Read the model definition and answer for the solid it produces. Units are mm, in the model's axes. Face numbers are marked on the shaded views. A direction names the side the tool comes from. Give positions to 0.01 mm unless a question says otherwise; leave off trailing zeros. Loops run counter-clockwise (first coordinate to the right, second up) from the corner with the lowest first, then second, coordinate; pieces in that order, holes last. Notation, with made-up numbers: (47.25, 20) -> (86.25, 20) arc R24 cw to (86.25, 46) -> close; hole circle Ø9 at (66.5, -2). An arc over 180 degrees is marked (long way). One line per item, written item: value. Start each with the question number.
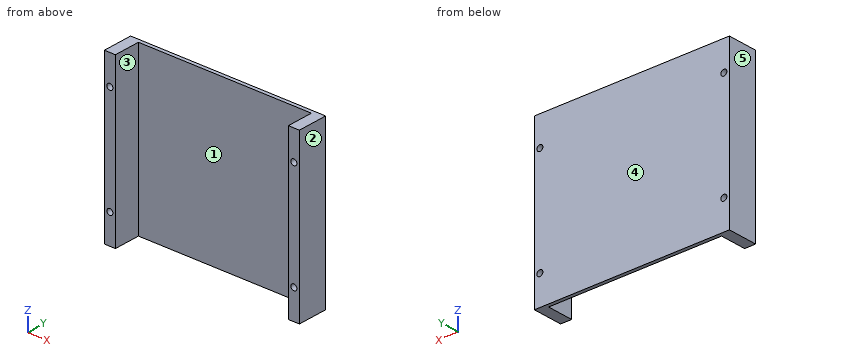
Autodesk Inventor part; units mm, degrees
ref_plane "YZ Plane" through (0, 0, 0) normal (1, 0, 0) x (0, 1, 0)
ref_plane "XZ Plane" through (0, 0, 0) normal (0, 1, 0) x (-1, 0, 0)
ref_plane "XY Plane" through (0, 0, 0) normal (0, 0, 1) x (1, 0, 0)
sketch "Sketch1" plane through (0, 0, 0) normal (0, 0, 1) x (1, 0, 0)
  line L0 (0, 26.035) -> (-84.1883, 26.035)
  line L1 (-84.1883, 26.035) -> (-84.1883, 0)
  line L2 (-84.1883, 0) -> (-74.6633, 0)
  line L3 (-74.6633, 0) -> (-74.6633, 22.86)
  line L4 (-74.6633, 22.86) -> (0, 22.86)
  line L5 (0, 0) -> (0, 26.035) construction
  line L6 (0, 26.035) -> (84.1883, 26.035)
  line L7 (84.1883, 26.035) -> (84.1883, 0)
  line L8 (84.1883, 0) -> (74.6633, 0)
  line L9 (74.6633, 0) -> (74.6633, 22.86)
  line L10 (74.6633, 22.86) -> (0, 22.86)
  dimension "d0" = 22.86
  dimension "d1" = 3.175
  dimension "d2" = 9.525
  dimension "d3" = 74.6633
extrude "Extrusion1" add sketch "Sketch1" along normal mid plane 143.1798
sketch "Sketch2" plane through (-84.1883, 0, 71.5899) normal (0, -1, 0) x (1, 0, 0)
  line L0 (0, -143.1798) -> (168.3766, -143.1798) construction
  line L1 (4.7625, -143.1798) -> (4.7625, -0.1575) construction
  line L2 (0, 0) -> (9.525, 0)
  point P0 (84.1883, -71.5899)
  point P1 (4.7625, -117.7798)
  point P2 (4.7625, -25.4)
  dimension "d6" = 4.7625
  dimension "d7" = 25.4
  dimension "d8" = 25.4
hole "Hole1" at (-79.4258, 0, -46.1899) at (-79.4258, 0, 46.1899) direction (0, 1, 0) diameter 5.1054 end through all
mirror "Mirror1" about plane through (0, 0, 0) normal (1, 0, 0) of "Hole1"
sketch "Sketch3" plane through (-84.1883, 26.035, 71.5899) normal (0, 1, 0) x (1, 0, 0)
  line L0 (11.1125, 0) -> (157.2641, 0) construction
  line L1 (157.2641, 0) -> (157.2641, 143.1798) construction
  line L2 (157.2641, 143.1798) -> (11.1125, 143.1798) construction
  line L3 (11.1125, 143.1798) -> (11.1125, 0) construction
  line L4 (11.1125, 0) -> (157.2641, 143.1798) construction
  line L5 (157.2641, 0) -> (11.1125, 143.1798) construction
  line L6 (51.9303, 1.2954) -> (83.4263, 1.2954)
  line L7 (83.4263, 1.2954) -> (83.4263, 9.9314)
  line L8 (83.4263, 9.9314) -> (51.9303, 9.9314)
  line L9 (51.9303, 9.9314) -> (51.9303, 1.2954)
  line L10 (51.9303, 1.2954) -> (83.4263, 9.9314) construction
  line L11 (83.4263, 1.2954) -> (51.9303, 9.9314) construction
  line L12 (168.3766, 0) -> (0, 0)
  line L13 (84.9503, 1.2954) -> (116.4463, 1.2954)
  line L14 (116.4463, 1.2954) -> (116.4463, 9.9314)
  line L15 (116.4463, 9.9314) -> (84.9503, 9.9314)
  line L16 (84.9503, 9.9314) -> (84.9503, 1.2954)
  line L17 (84.9503, 1.2954) -> (116.4463, 9.9314) construction
  line L18 (116.4463, 1.2954) -> (84.9503, 9.9314) construction
  line L19 (123.5075, 2.8702) -> (145.4785, 2.8702)
  line L20 (145.4785, 2.8702) -> (145.4785, 20.6502)
  line L21 (145.4785, 20.6502) -> (123.5075, 20.6502)
  line L22 (123.5075, 20.6502) -> (123.5075, 2.8702)
  line L23 (123.5075, 2.8702) -> (145.4785, 20.6502) construction
  line L24 (145.4785, 2.8702) -> (123.5075, 20.6502) construction
  line L25 (15.2273, 15.1892) -> (24.7523, 15.1892)
  line L26 (24.7523, 15.1892) -> (24.7523, 92.4052)
  line L27 (24.7523, 92.4052) -> (15.2273, 92.4052)
  line L28 (15.2273, 92.4052) -> (15.2273, 15.1892)
  line L29 (15.2273, 15.1892) -> (24.7523, 92.4052) construction
  line L30 (24.7523, 15.1892) -> (15.2273, 92.4052) construction
  line L31 (123.0503, 118.7704) -> (133.0833, 118.7704)
  line L32 (133.0833, 118.7704) -> (133.0833, 140.8684)
  line L33 (133.0833, 140.8684) -> (123.0503, 140.8684)
  line L34 (123.0503, 140.8684) -> (123.0503, 118.7704)
  line L35 (123.0503, 118.7704) -> (133.0833, 140.8684) construction
  line L36 (133.0833, 118.7704) -> (123.0503, 140.8684) construction
  line L37 (137.5791, 97.028) -> (157.2641, 97.028)
  line L38 (157.2641, 97.028) -> (157.2641, 133.096)
  line L39 (157.2641, 133.096) -> (137.5791, 133.096)
  line L40 (137.5791, 133.096) -> (137.5791, 97.028)
  line L41 (137.5791, 97.028) -> (157.2641, 133.096) construction
  line L42 (157.2641, 97.028) -> (137.5791, 133.096) construction
  line L43 (144.5133, 16.3322) -> (154.0383, 16.3322)
  line L44 (154.0383, 16.3322) -> (154.0383, 95.4786)
  line L45 (154.0383, 95.4786) -> (144.5133, 95.4786)
  line L46 (144.5133, 95.4786) -> (144.5133, 16.3322)
  line L47 (144.5133, 16.3322) -> (154.0383, 95.4786) construction
  line L48 (154.0383, 16.3322) -> (144.5133, 95.4786) construction
  line L49 (36.8173, 121.8184) -> (48.1203, 121.8184)
  line L50 (48.1203, 121.8184) -> (48.1203, 139.0904)
  line L51 (48.1203, 139.0904) -> (36.8173, 139.0904)
  line L52 (36.8173, 139.0904) -> (36.8173, 121.8184)
  line L53 (36.8173, 121.8184) -> (48.1203, 139.0904) construction
  line L54 (48.1203, 121.8184) -> (36.8173, 139.0904) construction
  line L55 (29.0703, 4.1148) -> (37.8333, 4.1148)
  line L56 (37.8333, 4.1148) -> (37.8333, 12.8778)
  line L57 (37.8333, 12.8778) -> (29.0703, 12.8778)
  line L58 (29.0703, 12.8778) -> (29.0703, 4.1148)
  line L59 (29.0703, 4.1148) -> (37.8333, 12.8778) construction
  line L60 (37.8333, 4.1148) -> (29.0703, 12.8778) construction
  line L61 (15.2273, 95.2754) -> (24.7523, 95.2754)
  line L62 (24.7523, 95.2754) -> (24.7523, 104.8004)
  line L63 (24.7523, 104.8004) -> (15.2273, 104.8004)
  line L64 (15.2273, 104.8004) -> (15.2273, 95.2754)
  line L65 (15.2273, 95.2754) -> (24.7523, 104.8004) construction
  line L66 (24.7523, 95.2754) -> (15.2273, 104.8004) construction
  line L67 (15.2273, 106.68) -> (25.8953, 106.68)
  line L68 (25.8953, 106.68) -> (25.8953, 114.681)
  line L69 (25.8953, 114.681) -> (15.2273, 114.681)
  line L70 (15.2273, 114.681) -> (15.2273, 106.68)
  line L71 (15.2273, 106.68) -> (25.8953, 114.681) construction
  line L72 (25.8953, 106.68) -> (15.2273, 114.681) construction
  point P0 (84.1883, 71.5899)
  point P1 (67.6783, 5.6134)
  point P2 (100.6983, 5.6134)
  point P3 (134.493, 11.7602)
  point P4 (19.9898, 53.7972)
  point P5 (128.0668, 129.8194)
  point P6 (147.4216, 115.062)
  point P7 (149.2758, 55.9054)
  point P8 (42.4688, 130.4544)
  point P9 (33.4518, 8.4963)
  point P10 (19.9898, 100.0379)
  point P11 (20.5613, 110.6805)
  dimension "d16" = 143.1798
  dimension "d17" = 146.1516
  dimension "d18" = 31.496
  dimension "d19" = 8.636
  dimension "d20" = 40.8178
  dimension "d21" = 1.2954
  dimension "d22" = 31.496
  dimension "d23" = 8.636
  dimension "d24" = 73.8378
  dimension "d25" = 1.2954
  dimension "d26" = 17.78
  dimension "d27" = 21.971
  dimension "d28" = 2.8702
  dimension "d29" = 112.395
  dimension "d30" = 77.216
  dimension "d31" = 9.525
  dimension "d32" = 15.1892
  dimension "d33" = 4.1148
  dimension "d34" = 10.033
  dimension "d35" = 22.098
  dimension "d36" = 111.9378
  dimension "d37" = 118.7704
  dimension "d38" = 19.685
  dimension "d39" = 36.068
  dimension "d40" = 97.028
  dimension "d41" = 9.525
  dimension "d42" = 79.1464
  dimension "d43" = 16.3322
  dimension "d44" = 133.4008
  dimension "d45" = 11.303
  dimension "d46" = 17.272
  dimension "d47" = 25.7048
  dimension "d48" = 121.8184
  dimension "d49" = 8.763
  dimension "d50" = 8.763
  dimension "d51" = 17.9578
  dimension "d52" = 4.1148
  dimension "d53" = 9.525
  dimension "d54" = 9.525
  dimension "d55" = 95.2754
  dimension "d56" = 4.1148
  dimension "d57" = 10.668
  dimension "d58" = 8.001
  dimension "d59" = 4.1148
  dimension "d60" = 106.68
equation "\"d0\" = heightForRIO"
equation "\"d1\" = topWallThickness"
equation "\"d2\" = edgeWallThickness"
equation "\"d3\" = 0.5 * widthOfRIO + widthAirGap"
equation "\"d4\" = depthOfRIO"
equation "\"d6\" = 0.5 * edgeWallThickness"
equation "\"d16\" = depthOfRIO"
equation "\"d17\" = widthOfRIO"
equation "\"d18\" = widthForBottomRelay"
equation "\"d19\" = depthForBottomRelay"
equation "\"d20\" = edgeToBottomRelay"
equation "\"d21\" = bottomToBottomRelay"
equation "\"d22\" = widthForBottomAnalogIn"
equation "\"d23\" = depthForBottomAnalogIn"
equation "\"d24\" = edgeToBottomAnalogIn"
equation "\"d25\" = bottomToBottomAnalogIn"
equation "\"d26\" = buttonDepth"
equation "\"d27\" = buttonWidth"
equation "\"d28\" = bottomToBottomButton"
equation "\"d29\" = edgeToBottomButton"
equation "\"d30\" = depthLeftDIO"
equation "\"d31\" = widthLeftDIO"
equation "\"d32\" = bottomToLeftDIO"
equation "\"d33\" = edgeToLeftDIO"
equation "\"d34\" = widthSPI"
equation "\"d35\" = depthSPI"
equation "\"d36\" = edgeToSPI"
equation "\"d37\" = bottomToSPI"
equation "\"d38\" = widthLight"
equation "\"d39\" = depthLight"
equation "\"d40\" = bottomToLight"
equation "\"d41\" = widthPWM"
equation "\"d42\" = depthPWM"
equation "\"d43\" = bottomToPWM"
equation "\"d44\" = edgeToPWM"
equation "\"d45\" = widthPower"
equation "\"d46\" = depthPower"
equation "\"d47\" = edgeToPower"
equation "\"d48\" = bottomToPower"
equation "\"d49\" = widthRSL"
equation "\"d50\" = depthRSL"
equation "\"d51\" = edgeToRSL"
equation "\"d52\" = bottomToRSL"
equation "\"d53\" = widthRS232"
equation "\"d54\" = depthRS232"
equation "\"d55\" = bottomToRS232"
equation "\"d56\" = edgeToRS232"
equation "\"d57\" = widthI2C"
equation "\"d58\" = depthI2C"
equation "\"d59\" = edgeToI2C"
equation "\"d60\" = bottomToI2C"
equation "\"heightForRIO\" = 22.86"
equation "\"topWallThickness\" = 3.175"
equation "\"edgeWallThickness\" = 9.525"
equation "\"widthOfRIO\" = 146.1516"
equation "\"widthAirGap\" = 1.5875"
equation "\"depthOfRIO\" = 143.1798"
equation "\"depthForBottomRelay\" = 8.636"
equation "\"widthForBottomRelay\" = 31.496"
equation "\"componentGap\" = 3.175"
equation "\"edgeToBottomRelay\" = 40.8178"
equation "\"bottomToBottomRelay\" = 1.2954"
equation "\"depthForBottomAnalogIn\" = 8.636"
equation "\"widthForBottomAnalogIn\" = 31.496"
equation "\"edgeToBottomAnalogIn\" = 73.8378"
equation "\"bottomToBottomAnalogIn\" = 1.2954"
equation "\"buttonWidth\" = 21.971"
equation "\"buttonDepth\" = 17.78"
equation "\"bottomToBottomButton\" = 2.8702"
equation "\"edgeToBottomButton\" = 112.395"
equation "\"widthLeftDIO\" = 9.525"
equation "\"depthLeftDIO\" = 77.216"
equation "\"bottomToLeftDIO\" = 15.1892"
equation "\"edgeToLeftDIO\" = 4.1148"
equation "\"widthSPI\" = 10.033"
equation "\"depthSPI\" = 22.098"
equation "\"edgeToSPI\" = 111.9378"
equation "\"bottomToSPI\" = 118.7704"
equation "\"widthLight\" = 19.685"
equation "\"depthLight\" = 36.068"
equation "\"bottomToLight\" = 97.028"
equation "\"widthPWM\" = 9.525"
equation "\"depthPWM\" = 79.1464"
equation "\"bottomToPWM\" = 16.3322"
equation "\"edgeToPWM\" = 133.4008"
equation "\"widthPower\" = 11.303"
equation "\"depthPower\" = 17.272"
equation "\"edgeToPower\" = 25.7048"
equation "\"bottomToPower\" = 121.8184"
equation "\"widthRSL\" = 8.763"
equation "\"depthRSL\" = 8.763"
equation "\"bottomToRSL\" = 4.1148"
equation "\"edgeToRSL\" = 17.9578"
equation "\"widthRS232\" = 9.525"
equation "\"depthRS232\" = 9.525"
equation "\"bottomToRS232\" = 95.2754"
equation "\"edgeToRS232\" = 4.1148"
equation "\"widthI2C\" = 10.668"
equation "\"depthI2C\" = 8.001"
equation "\"edgeToI2C\" = 4.1148"
equation "\"bottomToI2C\" = 106.68"
properties part number "RioCoverPlate"
Item 1: Section A-A, the plane y = 19.75 is taken. Determine the outline of the cut face in (x, z), plus the area to 3 significant figures.
Item 2: Consider L1, parallel to X at y = 7.75, z = -46.5; L2, parallel to X at y = 20.25, z = 56; L3, parallel to X at y = 17.5, z = -47.5. Determine where each line is inside the solid, lowest interval first. Write a range as [from, to].
Item 3: Section C-C, the plane x = 33 is taken. Determine the outline of the cut face in (y, z) (3 decimals).
Item 4: Flat-ended cylindrical pins translate along their axes: pin 1 (1 mm diameter, centred on x = -40, z = 19.5, fed in from -Y); pin 2 (12 mm diameter, centred on x = 6.5, y = 18.5, fed in from -Z); pin 3 (4.5 mm diameter, centred on x = -79.43, z = 46.19, fed in from +Y). Find the tip coordinate at first contact, or state that the pin passes through.
Item 5: For the marked faces 1 and 2, determine the directions among +Z, -Z, +X, -X, +Y, -Y from which every point of the face is accessible in a straight line to the end or side of a thin tool.
Item 6: Determine the mould class of the marked faces 3, 4 and 5 for opening direction X: pulls with the +X half, pulls with the -X half, needs draft (parallel to the pull), parting line crosses it, or undercut.
Item 7: Section B-B, the plane z = -9.5 is taken. Determine the outline of the cut face in (x, y) (3 decimals).
Computed values:
1. outline: (-84.19, -71.59) -> (-74.66, -71.59) -> (-74.66, 71.59) -> (-84.19, 71.59) -> close; (74.66, -71.59) -> (84.19, -71.59) -> (84.19, 71.59) -> (74.66, 71.59) -> close; hole circle Ø5.11 at (-79.43, -46.19); hole circle Ø5.11 at (-79.43, 46.19); hole circle Ø5.11 at (79.43, -46.19); hole circle Ø5.11 at (79.43, 46.19)
1. area: 2,650 mm²
2. L1: [-84.19, -81.96], [-76.89, -74.66], [74.66, 76.89], [81.96, 84.19]
2. L2: [-84.19, -74.66], [74.66, 84.19]
2. L3: [-84.19, -81.62], [-77.23, -74.66], [74.66, 77.23], [81.62, 84.19]
3. outline: (22.86, -71.59) -> (26.035, -71.59) -> (26.035, 71.59) -> (22.86, 71.59) -> close
4. pin 1: y = 22.86
4. pin 2: z = -71.59
4. pin 3: through
5. face 1: +Z, -Z, -Y
5. face 2: +Z, -Z, +X, +Y, -Y
6. face 3: undercut
6. face 4: needs draft
6. face 5: pulls with the -X half
7. outline: (-84.188, 0) -> (-74.663, 0) -> (-74.663, 22.86) -> (74.663, 22.86) -> (74.663, 0) -> (84.188, 0) -> (84.188, 26.035) -> (-84.188, 26.035) -> close
